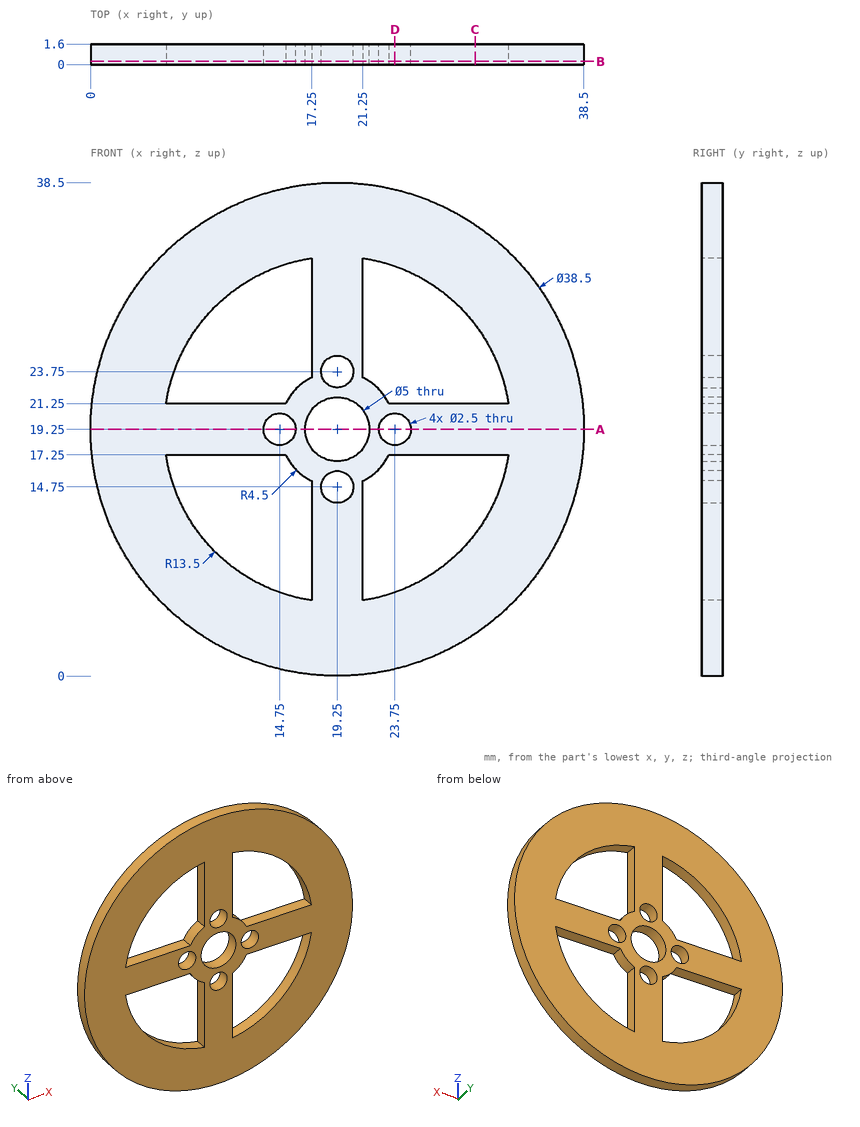
Study the drawing (mm; zero at the part's minimum x, y, z) and answer. Round coordinates to 2 decimals unless told otherwise and drop trailing zeros. Write each loop counter-clockwise with the first axis right and the second up, starting at its lowest first coordinate (ties: lowest second). Pieces come first, ordered by that corner, then holes.
Q1. Find section A-A on z = 19.25. Determine the outline of the cut face in (x, y), and give its area (3 significant figures).
Values:
outline: (0, 0) - (13.5, 0) - (13.5, 1.6) - (0, 1.6) - close; (16, 0) - (16.75, 0) - (16.75, 1.6) - (16, 1.6) - close; (21.75, 0) - (22.5, 0) - (22.5, 1.6) - (21.75, 1.6) - close; (25, 0) - (38.5, 0) - (38.5, 1.6) - (25, 1.6) - close
area: 45.6 mm2
Q2. Find section D-D on x = 23.75. Determine the outline of the cut face in (y, z).
Values:
outline: (0, 0.53) - (1.6, 0.53) - (1.6, 6.52) - (0, 6.52) - close; (0, 17.25) - (1.6, 17.25) - (1.6, 18) - (0, 18) - close; (0, 20.5) - (1.6, 20.5) - (1.6, 21.25) - (0, 21.25) - close; (0, 31.98) - (1.6, 31.98) - (1.6, 37.97) - (0, 37.97) - close
Q3. Find section C-C on x = 30. Determine the outline of the cut face in (y, z), and give its area (3 significant figures).
Values:
outline: (0, 3.28) - (1.6, 3.28) - (1.6, 11.08) - (0, 11.08) - close; (0, 17.25) - (1.6, 17.25) - (1.6, 21.25) - (0, 21.25) - close; (0, 27.42) - (1.6, 27.42) - (1.6, 35.22) - (0, 35.22) - close
area: 31.4 mm2
Q4. Straight lines are drawn through the part: line 1 (X direction, y = 1.1, z = 19.25); line 2 (X direction, y = 0.1, z = 24); line 3 (Z direction, x = 28.5, y = 0.5). For each, find the intervals that lie inside material, in ascending order.
Values:
line 1: x = 0 to 13.5, 16 to 16.75, 21.75 to 22.5, 25 to 38.5
line 2: x = 0.6 to 6.61, 17.25 to 18.03, 20.47 to 21.25, 31.89 to 37.9
line 3: z = 2.37 to 9.42, 17.25 to 21.25, 29.08 to 36.13
Q5. Find section B-B on y = 0.25. State how many separate pieces and enclosed holes the cut face has, and give its area (3 significant figures).
Values:
separate pieces: 1
enclosed holes: 9
area: 762 mm2
Q6. Flat-ended cylindrical pins translate along their axes: P1, Ø0.8, axis at x = 12.5, y = 0.5, coming from the -Z side; P2, Ø2, axis at x = 14.75, z = 19.25, coming from the -Y side; P3, Ø0.5, axis at y = 0.5, z = 30, coming from the +X side. Find the tip coordinate at first contact, or state that the pin passes through.
Values:
P1: stops at z = 1.08
P2: passes through
P3: stops at x = 35.38
